from build123d import *

# Parameters (mm, degrees)
EXTRUDE_1_DEPTH     = 6
SKETCH_2_R          = 1.5
CUT_EXTRUDE_1_DEPTH = 6
CUT_EXTRUDE_2_DEPTH = 2
SKETCH_4_R          = 35
CUT_EXTRUDE_3_DEPTH = 50.859803449


with BuildPart() as part:
    # Эскиз1 → Бобышка-Вытянуть1 (new body)
    with BuildSketch(Plane(origin=(0, 0, 0), x_dir=(1, 0, 0), z_dir=(0, 1, 0))):
        with BuildLine():
            Line((15, -35), (-15, -35))
            ThreePointArc((-15, -35), (-29.142135624, -29.142135624), (-35, -15))
            Line((-35, -15), (-35, 15))
            ThreePointArc((-35, 15), (-29.142135624, 29.142135624), (-15, 35))
            Line((-15, 35), (15, 35))
            ThreePointArc((15, 35), (29.142135624, 29.142135624), (35, 15))
            Line((35, 15), (35, -15))
            ThreePointArc((35, -15), (29.142135624, -29.142135624), (15, -35))
        make_face()
    extrude(amount=EXTRUDE_1_DEPTH)

    # Эскиз2 → Вырез-Вытянуть1 (cut)
    with BuildSketch(Plane(origin=(0, 0, 0), x_dir=(1, 0, 0), z_dir=(0, 1, 0))):
        with Locations(Location((-25, 25, 0), (0, 0, 270))):
            Circle(SKETCH_2_R)
        with Locations(Location((25, 25, 0), (0, 0, 270))):
            Circle(SKETCH_2_R)
        with Locations(Location((25, -25, 0), (0, 0, 270))):
            Circle(SKETCH_2_R)
        with Locations(Location((-25, -25, 0), (0, 0, 270))):
            Circle(SKETCH_2_R)
        with Locations(Location((0, 0, 0), (0, 0, 270))):
            Circle(SKETCH_2_R)
    extrude(amount=CUT_EXTRUDE_1_DEPTH, mode=Mode.SUBTRACT)

    # Эскиз3 → Вырез-Вытянуть2 (cut)
    with BuildSketch(Plane(origin=(0, 0, 0), x_dir=(1, 0, 0), z_dir=(0, 1, 0))):
        Polygon((-26.732050808, 28), (-28.464101615, 25), (-26.732050808, 22), (-23.267949192, 22), (-21.535898385, 25), (-23.267949192, 28), align=None)
        Polygon((23.267949192, 28), (21.535898385, 25), (23.267949192, 22), (26.732050808, 22), (28.464101615, 25), (26.732050808, 28), align=None)
        Polygon((23.267949192, -22), (21.535898385, -25), (23.267949192, -28), (26.732050808, -28), (28.464101615, -25), (26.732050808, -22), align=None)
        Polygon((-26.732050808, -22), (-28.464101615, -25), (-26.732050808, -28), (-23.267949192, -28), (-21.535898385, -25), (-23.267949192, -22), align=None)
        Polygon((-1.732050808, 3), (-3.464101615, 0), (-1.732050808, -3), (1.732050808, -3), (3.464101615, 0), (1.732050808, 3), align=None)
    extrude(amount=CUT_EXTRUDE_2_DEPTH, mode=Mode.SUBTRACT)

    # Эскиз4 → Вырез-Вытянуть3 (cut, through all)
    with BuildSketch(Plane(origin=(0, 0, 0), x_dir=(1, 0, 0), z_dir=(0, 1, 0))):
        with Locations((-66.622776602, 0)):
            Circle(SKETCH_4_R)
        with Locations((0, 66.622776602)):
            Circle(SKETCH_4_R)
        with Locations((66.622776602, 0)):
            Circle(SKETCH_4_R)
        with Locations((0, -66.622776602)):
            Circle(SKETCH_4_R)
    extrude(amount=CUT_EXTRUDE_3_DEPTH, mode=Mode.SUBTRACT)


solid = part.part
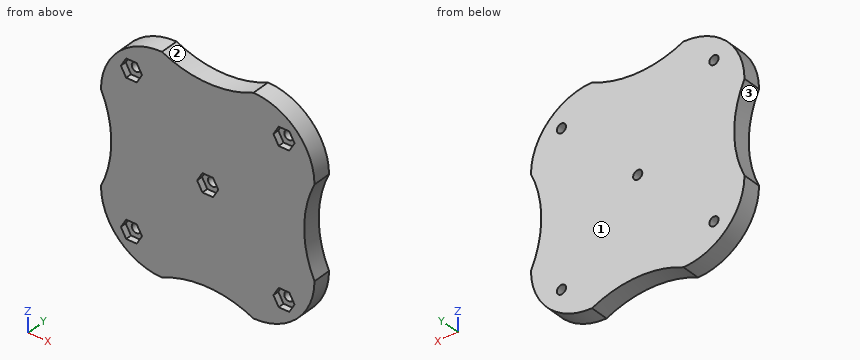
Could you check a few things on this model? Use its own coordinates, in mm. Face numbers are marked on the shaded views. Give positions to 0.01 mm unless a question says otherwise; leave off trailing zeros. Write each loop counter-clockwise with the first axis right and the second up, starting at its lowest first coordinate (ties: lowest second). Pieces come first, ordered by that corner, then holes. Notation, with made-up numbers: (62, 68.5) - (67, 68.5) arc R15 ccw to (67, 91.5) - close; hole circle Ø2 at (5.25, 61.25). An arc over 180 degrees is marked (long way). Use CSV: the item, a comma, the result in double quotes. Start each with the question number.
Item 1: I'm going to push flat-ended pins straight in: pin 1 (5 mm diameter, centred on x = 0, z = 0, fed in from -Y); pin 2 (1 mm diameter, centred on x = 0, y = 1, fed in from +Z); pin 3 (1 mm diameter, centred on x = 24.5, y = 1, fed in from -Z); pin 4 (2.5 mm diameter, centred on x = -25, z = -25, fed in from +Y). Where does each tip first touch, or does it pass through?
Item 2: I want a section at D-D, the plane z = 10. Please give me the cut outline in (x, y), then the cut area to 3 significant figures.
Item 3: I want a section at C-C, the plane x = 25. Please give me the cut outline in (y, z).
Item 4: If we mould it in two halves opening along Z, with no side actions, what happens to the marked faces 1, 2 and 3? For each: pulls with the +Z half, pulls with the -Z half, needs draft (parallel to the pull), parting line crosses it, or undercut.
Item 5: I want a section at B-B, the plane y = 5.1. Please give me the cut outline in (x, z).
Item 6: If I drill on line 1 along X through (y, z) = (5.1, 0); line 2 along Z through (x, y) = (25, 3), over which ranges is the centre line in solid material (lowest first)?
Item 7: I want a section at A-A, the plane x = 0. Please give me the cut outline in (y, z).
Findings:
1,pin 1,"stops at y = 2"
1,pin 2,"stops at z = 31.63"
1,pin 3,"stops at z = -32.86"
1,pin 4,"passes through"
2,outline,"(-33.08, 0) - (33.08, 0) - (33.08, 6) - (-33.08, 6) - close"
2,area,"397 mm2"
3,outline,"(0, -32.32) - (6, -32.32) - (6, -26.5) - (2, -26.5) - (2, -28) - (0, -28) - close; (0, -22) - (2, -22) - (2, -23.5) - (6, -23.5) - (6, 23.5) - (2, 23.5) - (2, 22) - (0, 22) - close; (0, 28) - (2, 28) - (2, 26.5) - (6, 26.5) - (6, 32.32) - (0, 32.32) - close"
4,face 1,"needs draft"
4,face 2,"pulls with the +Z half"
4,face 3,"undercut"
5,outline,"(-35, -15) arc R20 ccw to (-15, -35) arc R35 cw to (15, -35) arc R20 ccw to (35, -15) arc R35 cw to (35, 15) arc R20 ccw to (15, 35) arc R35 cw to (-15, 35) arc R20 ccw to (-35, 15) arc R35 cw to start; hole circle Ø3 at (-25, -25); hole circle Ø3 at (-25, 25); hole circle Ø3 at (0, 0); hole circle Ø3 at (25, -25); hole circle Ø3 at (25, 25)"
6,line 1,"x = -31.62 to -1.5, 1.5 to 31.62"
6,line 2,"z = -32.32 to -26.5, -23.5 to 23.5, 26.5 to 32.32"
7,outline,"(0, -31.62) - (6, -31.62) - (6, -1.5) - (2, -1.5) - (2, -3) - (0, -3) - close; (0, 3) - (2, 3) - (2, 1.5) - (6, 1.5) - (6, 31.62) - (0, 31.62) - close"
